Geometry check sheet. Reference: the model listing, model coordinates, mm. A direction names the side the tool comes from. Round coordinates to 2 decimals unless told otherwise and drop trailing zeros. Loops run counter-clockwise (first coordinate to the right, second up) from the corner with the lowest first, then second, coordinate; pieces in that order, holes last.
```python
from build123d import *

# Parameters (mm, degrees)
CYLINDER055_R            = 1
CYLINDER055_DEPTH        = 20
CYLINDER055_ROLL_ANGLE   = 90
CYLINDER054_R            = 5.5
CYLINDER054_DEPTH        = 20
CYLINDER054_ROLL_ANGLE   = 90
CLONE003_PLACEMENT_ANGLE = 90
PAD001_DEPTH             = 26.5
POCKET_DEPTH             = 21.001
SKETCH003_R              = 10.75
POCKET001_DEPTH          = 2.2
SKETCH004_R              = 1.75
POCKET002_DEPTH          = 4
SKETCH005_R              = 11
POCKET003_DEPTH          = 3.3
POCKET004_DEPTH          = 21.001


with BuildPart() as servo_horn_small_drill_master:
    # Cylinder055 → Cylinder055 (new body)
    with BuildSketch(Plane.XY):
        Circle(CYLINDER055_R)
    extrude(amount=CYLINDER055_DEPTH)


with BuildPart() as servo_horn_small_drill_master_1:
    # Cylinder055 roll: moved
    add(servo_horn_small_drill_master.part.rotate(Axis((0, 0, 0), (1, 0, 0)), CYLINDER055_ROLL_ANGLE))


with BuildPart() as servo_horn_small_drill_master_2:
    # Cylinder055 placement: moved
    add(servo_horn_small_drill_master_1.part.moved(Location((-3.5, 10, 7.5))))


with BuildPart() as clone002:
    # Clone002 base: copy of servo-horn-small-drill-master
    add(servo_horn_small_drill_master_2.part)


with BuildPart() as clone002_1:
    # Clone002 placement: moved
    add(clone002.part.moved(Location((0, -4e-06, -15.000002))))


with BuildPart() as servo_shaft_drill:
    # Cylinder054 → Cylinder054 (new body)
    with BuildSketch(Plane.XY):
        Circle(CYLINDER054_R)
    extrude(amount=CYLINDER054_DEPTH)


with BuildPart() as servo_shaft_drill_1:
    # Cylinder054 roll: moved
    add(servo_shaft_drill.part.rotate(Axis((0, 0, 0), (1, 0, 0)), CYLINDER054_ROLL_ANGLE))


with BuildPart() as servo_shaft_drill_2:
    # Cylinder054 placement: moved
    add(servo_shaft_drill_1.part.moved(Location((0, 10, 0))))


with BuildPart() as servo_drills_block1_master:
    # Clone001 base: copy of servo-horn-small-drill-master
    add(servo_horn_small_drill_master_2.part)


with BuildPart() as servo_drills_block1_master_1:
    # Clone001 placement: moved
    add(servo_drills_block1_master.part.moved(Location((10.85, -2e-06, -7.500002))))

    # Fusion041: union Clone002, servo-horn-small-drill-master, servo-shaft-drill
    add(clone002_1.part)
    add(servo_horn_small_drill_master_2.part)
    add(servo_shaft_drill_2.part)


with BuildPart() as clone_of_servo_drills_block1_master:
    # Clone003 base: copy of servo-Drills-block1-master
    add(servo_drills_block1_master_1.part)


with BuildPart() as clone_of_servo_drills_block1_master_1:
    # Clone003 placement: moved
    add(clone_of_servo_drills_block1_master.part.moved(Location((22, -49, 7e-06))).rotate(Axis((22, -49, 7e-06), (0, 0, 1)), CLONE003_PLACEMENT_ANGLE))


with BuildPart() as servo_horn_drills:
    # Fusion042 base: copy of servo-Drills-block1-master
    add(servo_drills_block1_master_1.part)

    # Fusion042: union Clone of servo-Drills-block1-master
    add(clone_of_servo_drills_block1_master_1.part)


with BuildPart() as leg:
    # Sketch001 → Pad001 (new body, symmetric)
    with BuildSketch(Plane.YZ):
        with BuildLine():
            Line((-49, 10.5), (0, 10.5))
            Line((0, 10.5), (0, -10.5))
            Line((0, -10.5), (-49, -10.5))
            ThreePointArc((-49, 10.5), (-59.5, 0), (-49, -10.5))
        make_face()
    extrude(amount=PAD001_DEPTH, both=True)

    # Sketch002 → Pocket (cut, through all)
    with BuildSketch(Plane(origin=(0, 0, 10.5), x_dir=(0, -1, 0), z_dir=(0, 0, 1))):
        Polygon((64, 21.5), (10, 21.5), (6, 17.5), (6, -19.5), (9, -22.5), (64, -22.5), align=None)
    extrude(amount=-POCKET_DEPTH, mode=Mode.SUBTRACT)

    # Sketch003 → Pocket001 (cut)
    with BuildSketch(Plane.YZ.offset(26.5)):
        with Locations((-49, 0)):
            Circle(SKETCH003_R)
    extrude(amount=-POCKET001_DEPTH, mode=Mode.SUBTRACT)

    # Sketch004 → Pocket002 (cut)
    with BuildSketch(Plane(origin=(-26.5, 0, 0), x_dir=(0, 1, 0), z_dir=(-1, 0, 0))):
        with Locations((-49, 0)):
            Circle(SKETCH004_R)
    extrude(amount=-POCKET002_DEPTH, mode=Mode.SUBTRACT)

    # Sketch005 → Pocket003 (cut)
    with BuildSketch(Plane(origin=(0, -6, 0), x_dir=(0, 0, -1), z_dir=(0, -1, 0))):
        Circle(SKETCH005_R)
    extrude(amount=-POCKET003_DEPTH, mode=Mode.SUBTRACT)

    # Sketch006 → Pocket004 (cut, through all)
    with BuildSketch(Plane(origin=(0, 0, 10.5), x_dir=(0, -1, 0), z_dir=(0, 0, 1))):
        Polygon((0, 18.5), (8, 26.5), (0, 26.5), align=None)
    extrude(amount=-POCKET004_DEPTH, mode=Mode.SUBTRACT)

    # Cut070: cut Servo-horn-drills
    add(servo_horn_drills.part, mode=Mode.SUBTRACT)


solid = leg.part
```
1) Access from +Z, -Z, +X, -X, +Y, -Y to the whole of each face (thin tool, end or side, straight path). Record for faces 5 (the face through (-5, -2.7, -5)), 6 (the face through (22.88, -42.387, 0.676)), 7 (the face through (19.5, -8, 0.1)), 8 (the face through (25.42, -38.25, -0.2)).
Report:
face 5: -Y
face 6: +X
face 7: +Z, -Z, -Y
face 8: +X, -Y
2) Sectioned sample at D-D, the plane y = -52.5. Record the cut outline in (x, z).
Report:
outline: (-26.5, -9.9) - (-22.5, -9.9) - (-22.5, 9.9) - (-26.5, 9.9) - close; (21.5, -9.9) - (24.3, -9.9) - (24.3, -8.5) - (21.5, -8.5) - close; (21.5, -6.5) - (24.3, -6.5) - (24.3, -4.24) - (21.5, -4.24) - close; (21.5, 4.24) - (24.3, 4.24) - (24.3, 6.5) - (21.5, 6.5) - close; (21.5, 8.5) - (24.3, 8.5) - (24.3, 9.9) - (21.5, 9.9) - close
3) Gauge pin test, flat ends, axial feed: pin 1 (12.5 mm diameter, centred on x = 0, z = 0, fed in from -Y); pin 2 (4 mm diameter, centred on y = -51, z = 5, fed in from +X); pin 3 (1.2 mm diameter, centred on x = -3.5, z = 7.5, fed in from +Y). Record the tip position at first contact, or that the pin passes through.
Report:
pin 1: stops at y = -2.7
pin 2: stops at x = 24.3
pin 3: passes through
4) Scan lines: line 1 along Z through (x, y) = (-25.45, -49); line 2 along X through (y, z) = (-48.5, 8.25); line 3 along X through (y, z) = (-30, 5). Record each from-to range of solid material in increasing order.
Report:
line 1: z = -10.5 to -1.75, 1.75 to 10.5
line 2: x = -26.5 to -22.5, 21.5 to 24.3
line 3: x = -26.5 to -22.5, 21.5 to 26.5
5) Sectioned sample at B-B, the plane y = -37. Record the cut outline in (x, z).
Report:
outline: (-26.5, -10.5) - (-22.5, -10.5) - (-22.5, 10.5) - (-26.5, 10.5) - close; (21.5, -10.5) - (26.5, -10.5) - (26.5, 10.5) - (21.5, 10.5) - close
6) Sectioned sample at C-C, the plane z = -4.5. Record the cut outline in (x, y), then the cut area to 4 significant figures.
Report:
outline: (-26.5, -58.49) - (-22.5, -58.49) - (-22.5, -9) - (-19.5, -6) - (-10.04, -6) - (-10.04, -2.7) - (-3.16, -2.7) - (-3.16, 0) - (-26.5, 0) - close; (3.16, -2.7) - (10.04, -2.7) - (10.04, -6) - (17.5, -6) - (21.5, -10) - (21.5, -45.84) - (24.3, -45.84) - (24.3, -39.24) - (26.5, -39.24) - (26.5, -8) - (18.5, 0) - (3.16, 0) - close; (21.5, -58.49) - (24.3, -58.49) - (24.3, -52.16) - (21.5, -52.16) - close
area: 627.5 mm2
7) Mould release check, pull along X, two halves, no side actions. Record for faces 1 (the face through (6, -5, 10.5)), 2 (the face through (-22.5, -34, 0)), 3 (the face through (24.3, -44, -5)), 4 (the face through (11, -4, 0)): +X half, -X half, draft (parallel to the pull), parting line (faces both ways), or undercut.
Report:
face 1: draft
face 2: undercut
face 3: +X half
face 4: undercut
8) Sectioned sample at A-A, the plane x = 0. Record the cut outline in (y, z), then the cut area to 3 significant figures.
Report:
outline: (-2.7, -10.5) - (0, -10.5) - (0, -5.5) - (-2.7, -5.5) - close; (-2.7, 5.5) - (0, 5.5) - (0, 10.5) - (-2.7, 10.5) - close
area: 27.0 mm2
